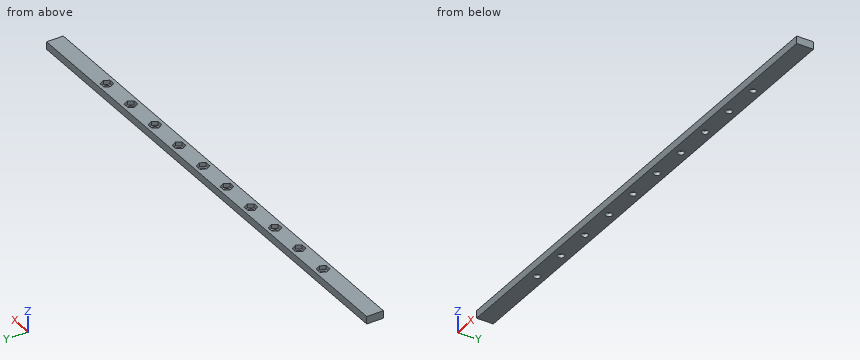
from build123d import *

# Parameters (mm, degrees)
SKETCH2_W                        = 200
SKETCH2_H                        = 6.65
BOSS_EXTRUDE1_DEPTH              = 3
CUT_EXTRUDE1_DEPTH               = 1.6
LPATTERN1_COUNT                  = 5
LPATTERN1_PITCH                  = 15
LPATTERN1_COUNT_DIR2             = 5
LPATTERN1_PITCH_DIR2             = 15
TALADRO_DE_MARGEN_PARA_M21_D     = 2.6
TALADRO_DE_MARGEN_PARA_M21_DEPTH = 12.5
TALADRO_DE_MARGEN_PARA_M21_TIP   = 0.781118805


with BuildPart() as part:
    # Sketch2 → Boss-Extrude1 (new body)
    with BuildSketch(Plane.XY):
        Rectangle(SKETCH2_W, SKETCH2_H)
    extrude(amount=BOSS_EXTRUDE1_DEPTH)

    # Sketch3 → Cut-Extrude1 (cut)
    with BuildSketch(Plane.XY.offset(3)):
        Polygon((-5.190598923, 0), (-6.345299462, 2), (-8.654700538, 2), (-9.809401077, 0), (-8.654700538, -2), (-6.345299462, -2), align=None)
        Polygon((5.190598923, 0), (6.345299462, 2), (8.654700538, 2), (9.809401077, 0), (8.654700538, -2), (6.345299462, -2), align=None)
    cut_extrude1 = extrude(amount=-CUT_EXTRUDE1_DEPTH, mode=Mode.SUBTRACT)

    # LPattern1: Cut-Extrude1 5 × 5
    with Locations(*[Vector(-1, 0, 0) * (i * LPATTERN1_PITCH) + Vector(1, 0, 0) * (j * LPATTERN1_PITCH_DIR2) for i in range(LPATTERN1_COUNT) for j in range(LPATTERN1_COUNT_DIR2) if (i, j) != (0, 0)]):
        add(cut_extrude1, mode=Mode.SUBTRACT)

    # Taladro de margen para M21
    with Locations(Plane.XY.offset(3)):
        with Locations((37.5, 0), (52.5, 0), (67.5, 0), (22.5, 0), (7.5, 0), (-67.5, 0), (-52.5, 0), (-37.5, 0), (-7.5, 0), (-22.5, 0)):
            Hole(TALADRO_DE_MARGEN_PARA_M21_D / 2, depth=TALADRO_DE_MARGEN_PARA_M21_DEPTH)
            with Locations((0, 0, -(TALADRO_DE_MARGEN_PARA_M21_DEPTH + TALADRO_DE_MARGEN_PARA_M21_TIP / 2))):  # 118° drill point
                Cone(0, TALADRO_DE_MARGEN_PARA_M21_D / 2, TALADRO_DE_MARGEN_PARA_M21_TIP, mode=Mode.SUBTRACT)


solid = part.part
Check sheet for the modelled part. Datum: model origin and axes. Units: mm. Round coordinates to 2 decimals unless told otherwise and drop trailing zeros. One line per question, with ' | ' between items. Start each with the question number.
Item 1: Scan lines: probe 1 along Y at (x, z) = (7.5, 1) (3 decimals); probe 2 along Y at (x, z) = (53.5, 1.1) (3 decimals). Record each from-to range of solid material in increasing order.
Item 2: Gauge pin test, flat end, axial feed: pin 1 Ø2 at (x, y) = (-53, -0.5) entering from +Z. Record the tip position at first contact, or that the pin passes through.
Item 3: Section check A-A (z = 2.55). State how many separate pieces and enclosed holes the cut face has, and give its area (3 significant figures).
Worked out:
1) probe 1: -3.325 to -1.3, 1.3 to 3.325 | probe 2: -3.325 to -0.831, 0.831 to 3.325
2) pin 1: z = 1.4
3) separate pieces: 1 | enclosed holes: 10 | area: 1,190 mm^2
